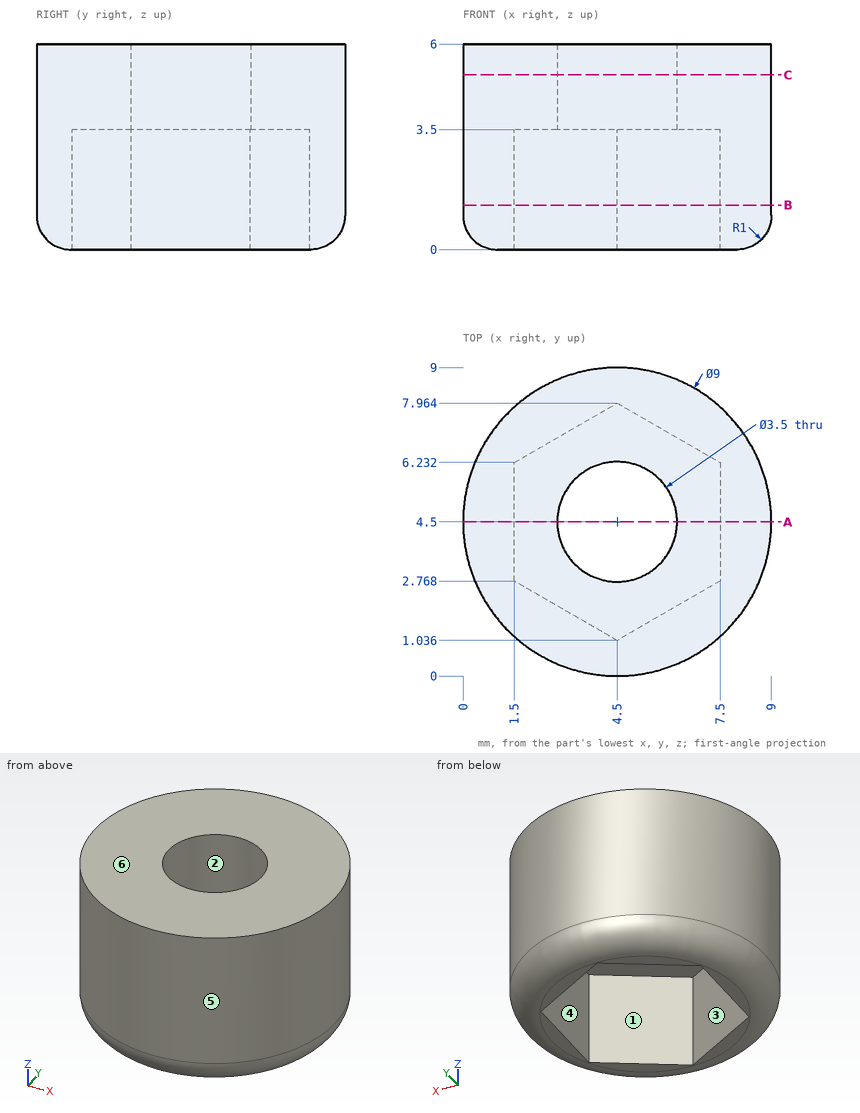
Here's the drawing with two shaded views (mm, measured from the low corner). I have some questions. A direction names the side the tool comes from. Round coordinates to 2 decimals unless told otherwise and drop trailing zeros. Loops run counter-clockwise (first coordinate to the right, second up) from the corner with the lowest first, then second, coordinate; pieces in that order, holes last. Notation, with made-up numbers: M -12,25.25 L 14,25.25 A31 ccw 14,52.25 Z; hole C -29.75,-9 d4. An arc over 180 degrees is marked long. Put each result on its own line as item: value.
Q1. I need wall thicknesses on probe 1 along Y at (x, z) = (4.5, 5.35); probe 2 along Z at (x, y) = (2.25, 5.5); probe 3 along Y at (x, z) = (7, 1.05). Which ranges of each line are inside material? Lowest first, please.
Check result:
probe 1: 0 to 2.75, 6.25 to 9
probe 2: 3.5 to 6
probe 3: 0.76 to 2.48, 6.52 to 8.24
Q2. On a 3-axis mill with a long thin cutter (end or side, diameter ignored), from which of +Z, -Z, +X, -X, +Y, -Y can I reach the whole of each face in a straight line? I mean the marked faces 1 and 2. Say none if no direction works.
Check result:
face 1: -Z
face 2: +Z, -Z
Q3. Thinking about a two-plate mould opening in Y: for the marked faces 3, 4, 5 and 6, which applies, released by +Y, released by -Y, zero draft, split by the parting line, or undercut?
Check result:
face 3: undercut
face 4: undercut
face 5: split by the parting line
face 6: zero draft
Q4. Imagine slicing it at B-B (z = 1.3). Write out the boundary of the cut face in (x, y), then the cut area to 3 significant figures.
Check result:
outline: C 4.5,4.5 d9; hole M 1.5,2.77 L 4.5,1.04 L 7.5,2.77 L 7.5,6.23 L 4.5,7.96 L 1.5,6.23 Z
area: 32.4 mm2
Q5. For pin 1 (1 mm diameter, centred on y = 5.5, z = 1, fed in from -X); pin 2 (1.5 mm diameter, centred on y = 8, z = 1, fed in from -X); pin 3 (3 mm diameter, centred on x = 2.5, z = 3, fed in from -Y), each with a flat end and sliding along its axis, tell me the tip position at first contact or that it passes through.
Check result:
pin 1: x = 0.03
pin 2: x = 0.94
pin 3: y = 0.03
Q6. Imagine slicing it at A-A (y = 4.5). Write out the boundary of the cut face in (x, z).
Check result:
outline: M 0,1 A1 ccw 1,0 L 1.5,0 L 1.5,3.5 L 2.75,3.5 L 2.75,6 L 0,6 Z; M 6.25,3.5 L 7.5,3.5 L 7.5,0 L 8,0 A1 ccw 9,1 L 9,6 L 6.25,6 Z
Q7. Imagine slicing it at C-C (z = 5.1). Write out the boundary of the cut face in (x, y).
Check result:
outline: C 4.5,4.5 d9; hole C 4.5,4.5 d3.5
